Autodesk Inventor part; units mm, degrees
ref_plane "YZ Plane" through (0, 0, 0) normal (1, 0, 0) x (0, 1, 0)
ref_plane "XZ Plane" through (0, 0, 0) normal (0, 1, 0) x (-1, 0, 0)
ref_plane "XY Plane" through (0, 0, 0) normal (0, 0, 1) x (1, 0, 0)
sketch "Sketch1" plane through (0, 0, 0) normal (0, 0, 1) x (1, 0, 0)
  circle A0 centre (0, 0) radius 3
  dimension "d0" = 6
extrude "Extrusion1" add sketch "Sketch1" along normal blind 90
sketch "Sketch2" plane through (0, 0, 90) normal (0, 0, 1) x (1, 0, 0)
  circle A0 centre (0, 0) radius 2
  circle A1 centre (0, 0) radius 3
  dimension "d3" = 4
extrude "Extrusion2" cut sketch "Sketch2" against normal blind 15
thread "Thread1"
fillet "Fillet1" radius 0.25 1 edges at (-2, 0, 90)
fillet "Fillet2" radius 1.5 1 edges at (-3, 0, 75)
chamfer "Chamfer1" distance 0.5 angle 45 1 edges at (-3, 0, 0)
properties part number "hridel_pro_kola" material "Iron, Cast"
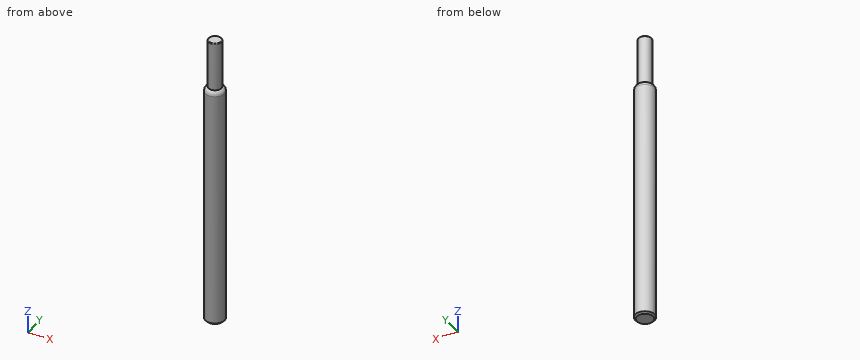
Source: CAD feature listing. Evaluate the final solid. Frame: model axes, mm. Give positions to 0.01 mm unless a question says otherwise; leave off trailing zeros. Write each loop counter-clockwise with the first axis right and the second up, starting at its lowest first coordinate (ties: lowest second). Pieces come first, ordered by that corner, then holes. Notation, with made-up numbers: (78, 1.25) - (94, 1.25) arc R14 ccw to (94, 17.25) - close; hole circle Ø8 at (3, 72.5). An arc over 180 degrees is marked (long way). One line per item, written item: value. Start each with the question number.
Q1. Section query A-A, the plane z = 69. Return the cut outline in (x, y), then the cut area to 3 significant figures.
Q2. Material intervals for probe 1 along Y at (x, z) = (2.25, 15); probe 2 along Y at (x, z) = (-0.25, 23.5); probe 3 along X at (y, z) = (0.5, 63), sorted ascending. Write a range as from..to.
Q3. First-contact query: pin 1 Ø1 at (x, z) = (-2, 48) entering from +Y. Flat tip, straight axial feed; report the tip coordinate or a pass-through.
Answer:
1. outline: circle Ø6 at (0, 0)
1. area: 28.3 mm2
2. probe 1: y = -1.98..1.98
2. probe 2: y = -2.99..2.99
2. probe 3: x = -2.96..2.96
3. pin 1: stops at y = 2.6
